Autodesk Inventor part; units mm, degrees
ref_plane "YZ Plane" through (0, 0, 0) normal (1, 0, 0) x (0, 1, 0)
ref_plane "XZ Plane" through (0, 0, 0) normal (0, 1, 0) x (-1, 0, 0)
ref_plane "XY Plane" through (0, 0, 0) normal (0, 0, 1) x (1, 0, 0)
sketch "Sketch1" plane through (0, 0, 0) normal (0, 1, 0) x (-1, 0, 0)
  circle A0 centre (0, 0) radius 6
  circle A1 centre (0, 0) radius 5
  dimension "d0" = 12
  dimension "d1" = 10
extrude "Extrusion1" add sketch "Sketch1" along normal blind 115 contours A0 | A1
extrude "Extrusion2" cut sketch "Sketch1" along normal blind 10
sketch "Sketch2" plane through (0, 115, 0) normal (0, 1, 0) x (1, 0, 0)
  circle A0 centre (0, 0) radius 5
  circle A1 centre (0, 0) radius 6
  dimension "d6" = 10
extrude "Extrusion3" cut sketch "Sketch2" against normal blind 10
thread "Thread1"
thread "Thread2"
properties part number "Handle" material "Stainless Steel"
Model file for the job. Use its own axes, mm. A direction names the side the tool comes from. Round coordinates to 2 decimals unless told otherwise and drop trailing zeros. Loops run counter-clockwise (first coordinate to the right, second up) from the corner with the lowest first, then second, coordinate; pieces in that order, holes last.
1. Band-saw the part on C-C, the plane y = 89.5. List the corners of the cut face in (x, z), and give its area (3 significant figures).
Check values:
outline: circle Ø12 at (0, 0)
area: 113 mm2
2. Band-saw the part on A-A, the plane x = 0. List the corners of the cut face in (y, z).
Check values:
outline: (0, -5) - (10, -5) - (10, -6) - (105, -6) - (105, -5) - (115, -5) - (115, 5) - (105, 5) - (105, 6) - (10, 6) - (10, 5) - (0, 5) - close
3. Band-saw the part on B-B, the plane z = 0. List the corners of the cut face in (x, y), and give its area (3 significant figures).
Check values:
outline: (-6, 10) - (-5, 10) - (-5, 0) - (5, 0) - (5, 10) - (6, 10) - (6, 105) - (5, 105) - (5, 115) - (-5, 115) - (-5, 105) - (-6, 105) - close
area: 1,340 mm2
4. Drop a flat-ended pin along its axis: P1, Ø4, axis at y = 20.5, z = -4.5, coming from the +X side. Give the stop position or say it passes through.
Check values:
P1: stops at x = 5.45
5. Wall check: probe 1 along Y at (x, z) = (-4.5, 3.5); probe 2 along Z at (x, y) = (-0.5, 68); probe 3 along Z at (x, y) = (3.75, 76). Give the ranges that are in metal, low to high.
Check values:
probe 1: y = 10 to 105
probe 2: z = -5.98 to 5.98
probe 3: z = -4.68 to 4.68
6. Tool access for faces 1 (the cylindrical face through (-1.08, 110.07, 4.88)), 2 (the flat face through (4, 10, 4)), 3 (the cylindrical face through (6, 57, 0)): list every direction of +Z, -Z, +X, -X, +Y, -Y with a clear straight run to the whole face (end or side of a thin tool).
Check values:
face 1: +Y
face 2: -Y
face 3: +Y, -Y
